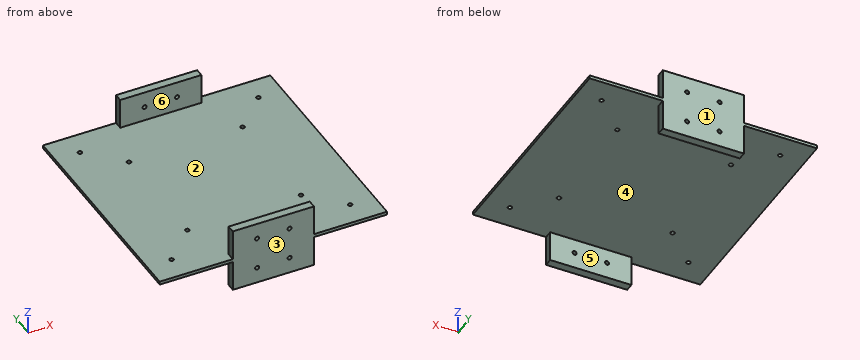
Autodesk Fusion 360 part; units mm, degrees
sketch "Sketch1" plane through (0, 0, 0) normal (0, 0, 1) x (1, 0, 0)
  line L0 (0, 0) -> (140, 0)
  line L1 (140, 0) -> (140, 140)
  line L2 (140, 140) -> (0, 140)
  line L3 (0, 140) -> (0, 0)
  dimension "d1" = 140
  dimension "d2" = 140
extrude "Extrude1" add sketch "Sketch1" along normal blind 2
sketch "Sketch2" plane through (0, 0, 2) normal (0, 0, 1) x (-1, 0, 0)
  line L0 (0, -140) -> (0, 0)
  line L1 (0, 0) -> (-140, 0)
  line L2 (-140, 0) -> (-140, -140)
  line L3 (-140, -140) -> (0, -140)
  line L4 (-45, 0) -> (-95, 0)
  line L5 (-95, 0) -> (-95, -5)
  line L6 (-95, -5) -> (-45, -5)
  line L7 (-45, -5) -> (-45, 0)
  line L8 (-45, -140) -> (-95, -140)
  line L9 (-95, -140) -> (-95, -135)
  line L10 (-95, -135) -> (-45, -135)
  line L11 (-45, -135) -> (-45, -140)
  dimension "d5" = 45
  dimension "d6" = 45
  dimension "d7" = 5
  dimension "d8" = 50
  dimension "d9" = 5
  dimension "d10" = 45
extrude "Extrude2" add sketch "Sketch2" along normal blind 19 and the other way blind 21 contours L3 L8 L9 L10 L11 | L1 L4 L5 L6 L7
sketch "Sketch3" plane through (0, 0, 0) normal (0, -1, 0) x (1, 0, 0)
  line L0 (45, 2) -> (0, 2)
  line L1 (0, 2) -> (0, 0)
  line L2 (0, 0) -> (45, 0)
  line L3 (45, 0) -> (45, -19)
  line L4 (45, -19) -> (95, -19)
  line L5 (95, -19) -> (95, 0)
  line L6 (95, 0) -> (140, 0)
  line L7 (140, 0) -> (140, 2)
  line L8 (140, 2) -> (95, 2)
  line L9 (95, 2) -> (95, 21)
  line L10 (95, 21) -> (45, 21)
  line L11 (45, 21) -> (45, 2)
  line L12 (60, -9) -> (80, -9) construction
  line L13 (80, -9) -> (80, 11) construction
  line L14 (80, 11) -> (60, 11) construction
  line L15 (60, 11) -> (60, -9) construction
  circle A0 centre (60, 11) radius 1.5
  circle A1 centre (80, 11) radius 1.5
  circle A2 centre (60, -9) radius 1.5
  circle A3 centre (80, -9) radius 1.5
  dimension "d15" = 20
  dimension "d16" = 20
  dimension "d17" = 10
  dimension "d18" = 15
  dimension "d19" = 3
  dimension "d20" = 3
  dimension "d21" = 3
  dimension "d22" = 3
hole "Hole1" at (60, 0, 11) at (80, 0, 11) at (60, 0, -9) at (80, 0, -9) direction (0, 1, 0) diameter 2.529 depth 140 tip angle 118
sketch "Sketch4" plane through (0, 0, 2) normal (0, 0, 1) x (-1, 0, 0)
  line L0 (-45, 0) -> (-45, -5)
  line L1 (-45, -5) -> (-95, -5)
  line L2 (-95, -5) -> (-95, 0)
  line L3 (-95, 0) -> (-140, 0)
  line L4 (-140, 0) -> (-140, -140)
  line L5 (-140, -140) -> (-95, -140)
  line L6 (-95, -140) -> (-95, -135)
  line L7 (-95, -135) -> (-45, -135)
  line L8 (-45, -135) -> (-45, -140)
  line L9 (-45, -140) -> (0, -140)
  line L10 (0, -140) -> (0, 0)
  line L11 (0, 0) -> (-45, 0)
  line L12 (-15, -15) -> (-125, -15) construction
  line L13 (-125, -15) -> (-125, -125) construction
  line L14 (-125, -125) -> (-15, -125) construction
  line L15 (-15, -125) -> (-15, -15) construction
  line L16 (-105, -35) -> (-105, -105) construction
  line L17 (-105, -105) -> (-35, -105) construction
  line L18 (-35, -105) -> (-35, -35) construction
  line L19 (-35, -35) -> (-105, -35) construction
  circle A0 centre (-15, -125) radius 1.5
  circle A1 centre (-125, -125) radius 1.5
  circle A2 centre (-35, -105) radius 1.5
  circle A3 centre (-105, -105) radius 1.5
  circle A4 centre (-105, -35) radius 1.5
  circle A5 centre (-35, -35) radius 1.5
  circle A6 centre (-15, -15) radius 1.5
  circle A7 centre (-125, -15) radius 1.5
  dimension "d28" = -20
  dimension "d29" = 3
  dimension "d30" = 3
  dimension "d31" = 3
  dimension "d32" = 3
  dimension "d33" = 3
  dimension "d34" = 3
  dimension "d35" = 3
  dimension "d36" = 3
hole "Hole2" at (15, 125, 2) at (125, 125, 2) at (105, 105, 2) at (35, 105, 2) at (35, 35, 2) at (125, 15, 2) at (105, 35, 2) at (15, 15, 2) direction (0, 0, -1) diameter 2.529 depth 2 tip angle 118
Geometry check sheet. Reference: the model listing, model coordinates, mm. Face numbers are marked on the shaded views. A direction names the side the tool comes from. Round coordinates to 2 decimals unless told otherwise and drop trailing zeros. Order: outer loops, then holes, each group sorted by start corner. A loop starts at its lowest first (then second) coordinate and runs counter-clockwise, first axis right, second up. Notation, with made-up numbers: M -34,-0.75 L 7,-0.75 A16 ccw 7,8.25 Z; hole C 9,84.25 d4. An arc over 180 degrees is marked long. Answer as CSV lines item,"result".
1) Tool access check on the marked faces 5 and 6. Record the directions out of +Z, -Z, +X, -X, +Y, -Y that give a thin tool (end or side, any length) a straight path to the whole face; none if there is none.
Entries:
face 5,"-Z, +X, -X"
face 6,"+Z, +X, -X"
2) Gauge pin test, flat ends, axial feed: pin 1 Ø2.5 at (y, z) = (138, -11.5) entering from -X; pin 2 Ø2 at (x, y) = (52.5, 125) entering from -Z; pin 3 Ø1.5 at (x, z) = (97, -9) entering from +Y; pin 4 Ø4 at (y, z) = (2, 14.5) entering from +X. Record the tip position at first contact, or that the pin passes through.
Entries:
pin 1,"x = 45"
pin 2,"z = 0"
pin 3,"through"
pin 4,"x = 95"
3) Sectioned sample at B-B on x = 68. Record the cut outline in (y, z), and give its area (3 significant figures).
Entries:
outline,"M 0,-19 L 5,-19 L 5,0 L 135,0 L 135,-19 L 140,-19 L 140,21 L 135,21 L 135,2 L 5,2 L 5,21 L 0,21 Z"
area,"660 mm2"
4) Sectioned sample at A-A on z = -14. Record the cut outline in (x, y).
Entries:
outline,"M 45,0 L 95,0 L 95,5 L 45,5 Z; M 45,135 L 95,135 L 95,140 L 45,140 Z"
5) Sectioned sample at C-C on y = 48.5. Record the cut outline in (x, z).
Entries:
outline,"M 0,0 L 140,0 L 140,2 L 0,2 Z"
6) Mould release check, pull along Y, two halves, no side actions. Record for the marked faces 1, 2, 3 and 4: +Y half, -Y half, draft (parallel to the pull), parting line (faces both ways), or undercut.
Entries:
face 1,"+Y half"
face 2,"undercut"
face 3,"-Y half"
face 4,"undercut"
7) Thickness scan on probe 1 along Z at (x, y) = (80, 2); probe 2 along X at (y, z) = (15, 1); probe 3 along Y at (x, z) = (105, 1). Record the ranges inside material, lowest first. Write a range as [from, to].
Entries:
probe 1,"[-19, -10.26], [-7.74, 9.74], [12.26, 21]"
probe 2,"[0, 13.74], [16.26, 123.74], [126.26, 140]"
probe 3,"[0, 33.74], [36.26, 103.74], [106.26, 140]"
